from build123d import *

# Parameters (mm, degrees)
SKETCH1_W                     = 76.2
SKETCH1_H                     = 914.4
BOSS_EXTRUDE1_DEPTH           = 3.175
SKETCH2_W                     = 3.556
SKETCH2_H                     = 12.954
CUT_EXTRUDE1_DEPTH            = 4.175
LPATTERN1_COUNT               = 2
LPATTERN1_PITCH               = 50.8
LPATTERN1_COPY_1_SKETCH_W     = 3.556
LPATTERN1_COPY_1_SKETCH_H     = 12.954
LPATTERN1_COPY_1_DEPTH        = 4.175
LPATTERN1_COL_COUNT           = 2
LPATTERN1_COL_PITCH           = 50.8
LPATTERN1_COL_COPY_1_SKETCH_W = 3.556
LPATTERN1_COL_COPY_1_SKETCH_H = 12.954
LPATTERN1_COL_COPY_1_DEPTH    = 4.175
SKETCH3_W                     = 3.556
SKETCH3_H                     = 12.954
CUT_EXTRUDE2_DEPTH            = 4.175
LPATTERN2_COUNT               = 2
LPATTERN2_PITCH               = 38.1
CUT_EXTRUDE3_DEPTH            = 4.175
SKETCH5_W                     = 76.2
SKETCH5_H                     = 44.45
BOSS_EXTRUDE2_DEPTH           = 3.175
SKETCH6_W                     = 41.275
SKETCH6_H                     = 19.05
CUT_EXTRUDE4_DEPTH            = 4.175
BOSS_EXTRUDE3_DEPTH           = 3.175
FILLET1_R                     = 25.4
F_8_CLEARANCE_HOLE1_D         = 4.4958


with BuildPart() as part:
    # Sketch1 → Boss-Extrude1 (new body)
    with BuildSketch(Plane(origin=(0, 0, 0), x_dir=(0, 0, -1), z_dir=(1, 0, 0))):
        Rectangle(SKETCH1_W, SKETCH1_H)
    extrude(amount=BOSS_EXTRUDE1_DEPTH)

    # Sketch2 → Cut-Extrude1 (cut, through all)
    with BuildSketch(Plane(origin=(3.175, 0, 0), x_dir=(0, 0, -1), z_dir=(1, 0, 0))):
        with Locations((5.499997, -211.0105)):
            Rectangle(SKETCH2_W, SKETCH2_H)
    cut_extrude1 = extrude(amount=-CUT_EXTRUDE1_DEPTH, mode=Mode.SUBTRACT)

    # Mirror1: Cut-Extrude1 across plane
    add(cut_extrude1.mirror(Plane.XY), mode=Mode.SUBTRACT)

    # LPattern1: Cut-Extrude1 ×2
    with Locations(*[(0, i * LPATTERN1_PITCH, 0) for i in range(1, LPATTERN1_COUNT)]):
        add(cut_extrude1, mode=Mode.SUBTRACT)

    # LPattern1 copy 1 sketch → LPattern1 copy 1 (cut, through all)
    with BuildSketch(Plane(origin=(3.175, 50.8, 0), x_dir=(0, 0, 1), z_dir=(1, 0, 0))):
        with Locations((5.499997, 211.0105)):
            Rectangle(LPATTERN1_COPY_1_SKETCH_W, LPATTERN1_COPY_1_SKETCH_H)
    extrude(amount=-LPATTERN1_COPY_1_DEPTH, mode=Mode.SUBTRACT)

    # LPattern1 col: Cut-Extrude1 ×2
    with Locations(*[(0, -i * LPATTERN1_COL_PITCH, 0) for i in range(1, LPATTERN1_COL_COUNT)]):
        add(cut_extrude1, mode=Mode.SUBTRACT)

    # LPattern1 col copy 1 sketch → LPattern1 col copy 1 (cut, through all)
    with BuildSketch(Plane(origin=(3.175, -50.8, 0), x_dir=(0, 0, 1), z_dir=(1, 0, 0))):
        with Locations((5.499997, 211.0105)):
            Rectangle(LPATTERN1_COL_COPY_1_SKETCH_W, LPATTERN1_COL_COPY_1_SKETCH_H)
    extrude(amount=-LPATTERN1_COL_COPY_1_DEPTH, mode=Mode.SUBTRACT)

    # Sketch3 → Cut-Extrude2 (cut, through all)
    with BuildSketch(Plane(origin=(3.175, 0, 0), x_dir=(0, 0, -1), z_dir=(1, 0, 0))):
        with Locations((5.499997, 128.7145)):
            Rectangle(SKETCH3_W, SKETCH3_H)
        with Locations((-5.499997, 128.7145)):
            Rectangle(SKETCH3_W, SKETCH3_H)
    cut_extrude2 = extrude(amount=-CUT_EXTRUDE2_DEPTH, mode=Mode.SUBTRACT)

    # LPattern2: Cut-Extrude2 ×2
    with Locations(*[(0, i * LPATTERN2_PITCH, 0) for i in range(1, LPATTERN2_COUNT)]):
        add(cut_extrude2, mode=Mode.SUBTRACT)

    # Sketch4 → Cut-Extrude3 (cut, through all)
    with BuildSketch(Plane(origin=(3.175, 0, 0), x_dir=(0, 0, -1), z_dir=(1, 0, 0))):
        Polygon((-38.1, 187.325), (0, 187.325), (38.1, 187.325), (38.1, 457.2), (-38.1, 457.2), align=None)
    extrude(amount=-CUT_EXTRUDE3_DEPTH, mode=Mode.SUBTRACT)

    # Sketch5 → Boss-Extrude2 (add)
    with BuildSketch(Plane(origin=(3.175, 0, 0), x_dir=(0, 0, -1), z_dir=(1, 0, 0))):
        with Locations((0, -479.425)):
            Rectangle(SKETCH5_W, SKETCH5_H)
    extrude(amount=-BOSS_EXTRUDE2_DEPTH)

    # Sketch6 → Cut-Extrude4 (cut, through all)
    with BuildSketch(Plane(origin=(3.175, 0, 0), x_dir=(0, 0, -1), z_dir=(1, 0, 0))):
        with Locations((0, 97.106805088)):
            Rectangle(SKETCH6_W, SKETCH6_H)
    extrude(amount=-CUT_EXTRUDE4_DEPTH, mode=Mode.SUBTRACT)

    # Sketch7 → Boss-Extrude3 (add)
    with BuildSketch(Plane(origin=(3.175, 0, 0), x_dir=(0, 0, -1), z_dir=(1, 0, 0))):
        Polygon((-76.2, -501.65), (76.2, -501.65), (76.2, -476.25), (38.1, -387.35), (-38.1, -387.35), (-76.2, -476.25), align=None)
    extrude(amount=-BOSS_EXTRUDE3_DEPTH)

    # Fillet1
    fillet1_edges = [part.edges().sort_by_distance(p)[0] for p in [
        (1.5875, -476.25, 76.2),
        (1.5875, -387.35, 38.1),
        (1.5875, -387.35, -38.1),
        (1.5875, -476.25, -76.2),
    ]]
    fillet(fillet1_edges, radius=FILLET1_R)

    # #8 Clearance Hole1 (through all)
    with Locations(Plane(origin=(3.175, 0, 0), x_dir=(0, 0, -1), z_dir=(1, 0, 0))):
        with Locations((-7.998961309, 41.861805088), (-28.953961309, 41.861805088), (20.6375, -18.825765594), (-20.6375, -18.825765594), (20.6375, -32.300765594), (-20.6375, -32.300765594), (-7.998961309, 114.251805088), (-28.953961309, 114.251805088)):
            Hole(F_8_CLEARANCE_HOLE1_D / 2)


solid = part.part
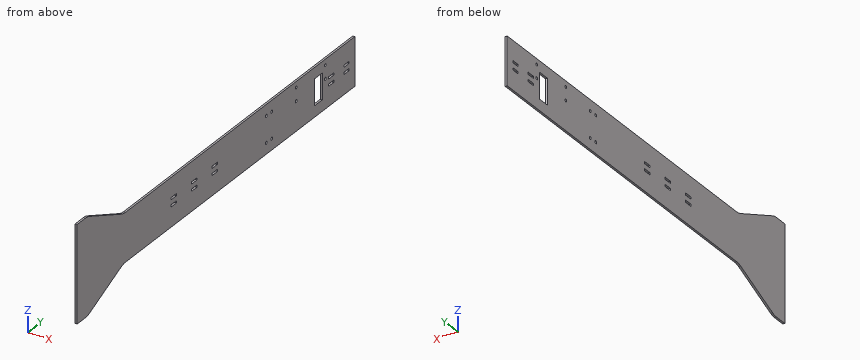
Input: part model. Units: mm. Frame: model coordinates. Give positions to 0.01 mm unless a question says otherwise; leave off trailing zeros. Order: outer loops, then holes, each group sorted by start corner. A loop starts at its lowest first (then second) coordinate and runs counter-clockwise, first axis right, second up. Notation, with made-up numbers: (-16.5, 31) -> (-7.5, 31) arc R23 cw to (-7.5, 54) -> close; hole circle Ø7 at (52, 39). An arc over 180 degrees is marked (long way). Use one line per item in the form item = value.
1) Section B-B, the plane z = -51. Return loops of the section in (x, y) (3 decimals), and give its area (3 significant figures).
Response values:
outline = (0, -501.65) -> (3.175, -501.65) -> (3.175, -417.45) -> (0, -417.45) -> close
area = 267 mm^2
2) First-contact query: pin 1 Ø1 at (x, y) = (1.5, 169.5) entering from -Z; pin 2 Ø1.6 at (x, y) = (1.5, 167.5) entering from +Z. Flat tips, straight axial feed; report the tip coordinate or a pass-through.
Response values:
pin_1 = -38.1
pin_2 = 38.1
3) Line query: probe 1 along Z at (x, y) = (2.8, -32); probe 2 along Z at (x, y) = (2.1, 114); probe 3 along Z at (x, y) = (2.55, 73). Output: solid intervals per line, ascending.
Response values:
probe_1 = -38.1 to -22.87, -18.41 to 18.41, 22.87 to 38.1
probe_2 = -38.1 to 5.77, 10.23 to 26.72, 31.19 to 38.1
probe_3 = -38.1 to 38.1
4) Section A-A, the plane y = 21.5. Return loops of the section in (x, z) (3 decimals), and give its area (3 significant figures).
Response values:
outline = (0, -38.1) -> (3.175, -38.1) -> (3.175, 38.1) -> (0, 38.1) -> close
area = 242 mm^2
5) Section C-C, the plane x = 0.9. Count the separate pieces of the cut face and the enclosed holes in it, and give its area (3 significant figures).
Response values:
separate_pieces = 1
enclosed_holes = 19
area = 56,400 mm^2
